Can you work these out from the drawing? Everything is in mm from the part's minimum corner. A direction names the side the tool comes from. Round coordinates to 2 decimals unless told otherwise and drop trailing zeros. Write each loop counter-clockwise with the first axis right and the second up, starting at its lowest first coordinate (ties: lowest second). Pieces come first, ordered by that corner, then holes. Notation, with made-up numbers: (42.5, 19) -> (94.5, 19) arc R6 cw to (94.5, 27) -> close; hole circle Ø3 at (-31, -20.5). An arc over 180 degrees is marked (long way). Put each result on its own line as item: value. Start each with the question number.
1. Suppose I cut it at C-C (z = 18.5). Please give me the cut outline in (x, y), then the cut area to 3 significant figures.
2. I need wall thicknesses on probe 1 along Z at (x, y) = (15, 36.25); probe 2 along X at (y, z) = (34.75, 15); probe 3 along Y at (x, z) = (20.75, 15.25). Which ranges of each line are inside material? Lowest first, please. Write a range as from..to.
3. Suppose I cut it at D-D (z = 6). Please give me the cut outline in (x, y).
4. Suppose I cut it at A-A (x = 15). Please give me the cut outline in (y, z), then the cut area to 3 significant figures.
5. Which directions (+Z, -Z, +X, -X, +Y, -Y) give clear straight access to the entire face, cutting with the end or side of a thin tool? Please do the marked faces 1 and 2.
6. Suppose I cut it at B-B (y = 5). Please give me the cut outline in (x, z), then the cut area to 3 significant figures.
7. For pin 1 (2 mm diameter, centred on y = 37.5, z = 21.5, fed in from -X) (1 decimal); pin 2 (3 mm diameter, centred on x = 6.5, y = 12, fed in from -Z); pin 3 (8 mm diameter, centred on y = 42.5, z = 4.5, fed in from +X), each with a flat end and sliding along its axis, tell me the tip position at first contact or that it passes through.
8. We'd pull the mould along Z, two halves only. Please class the marked faces 3, 4, 5 and 6: +Z half, -Z half, draft (parallel to the pull), parting line (faces both ways), or undercut.
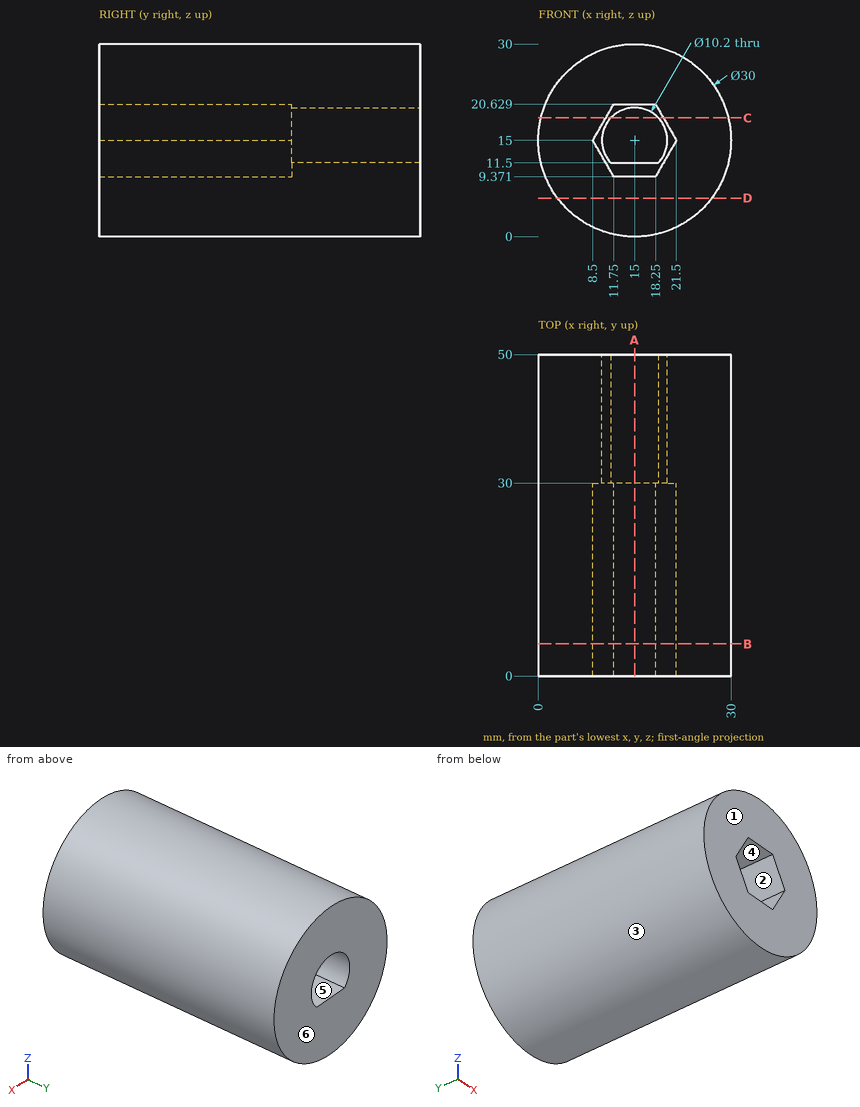
Verdict:
1. outline: (0.41, 0) -> (10.52, 0) -> (10.52, 30) -> (11.29, 30) -> (11.29, 50) -> (0.41, 50) -> close; (18.71, 30) -> (19.48, 30) -> (19.48, 0) -> (29.59, 0) -> (29.59, 50) -> (18.71, 50) -> close
1. area: 1,040 mm^2
2. probe 1: z = 0..11.5, 20.1..30
2. probe 2: x = 0..9.9, 20.1..30
2. probe 3: y = 30..50
3. outline: (3, 0) -> (27, 0) -> (27, 50) -> (3, 50) -> close
4. outline: (0, 0) -> (50, 0) -> (50, 11.5) -> (30, 11.5) -> (30, 9.37) -> (0, 9.37) -> close; (0, 20.63) -> (30, 20.63) -> (30, 20.1) -> (50, 20.1) -> (50, 30) -> (0, 30) -> close
4. area: 990 mm^2
5. face 1: +Z, -Z, +X, -X, -Y
5. face 2: -Y
6. outline: circle Ø30 at (15, 15); hole (8.5, 15) -> (11.75, 9.37) -> (18.25, 9.37) -> (21.5, 15) -> (18.25, 20.63) -> (11.75, 20.63) -> close
6. area: 597 mm^2
7. pin 1: stops at x = 1
7. pin 2: stops at z = 1.73
7. pin 3: stops at x = 28.52
8. face 3: parting line
8. face 4: undercut
8. face 5: undercut
8. face 6: draft
